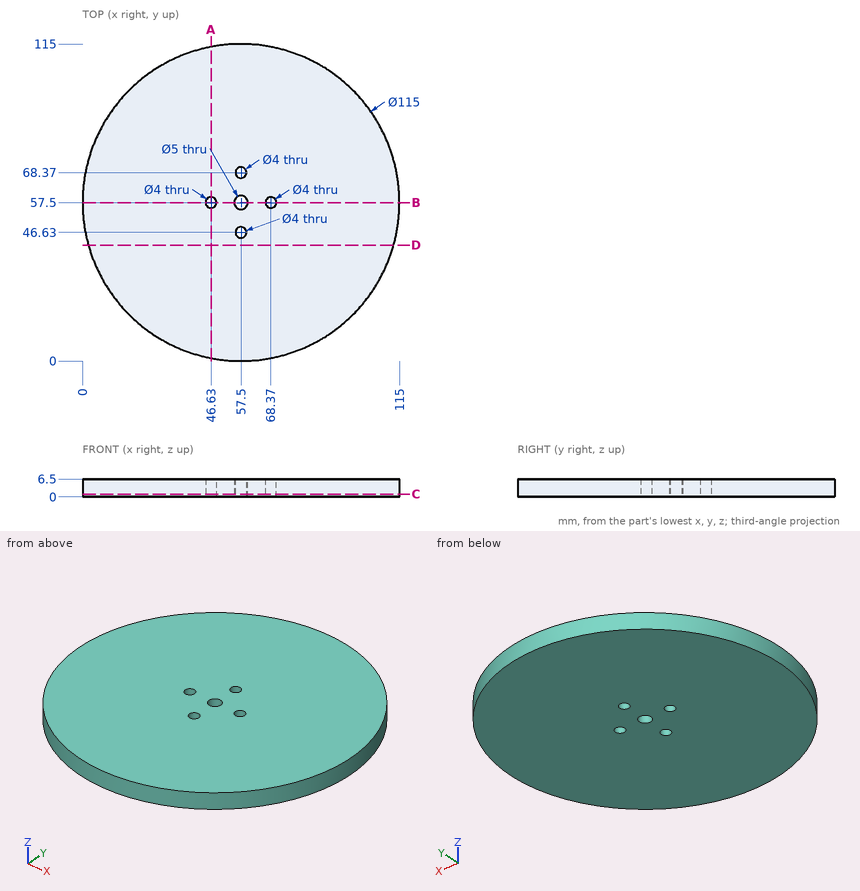
Job drawing, mm, ordinate dimensions from the low corner. One solid piece. Give positions to 0.01 mm unless a question says otherwise; leave off trailing zeros. Order: outer loops, then holes, each group sorted by start corner. A loop starts at its lowest first (then second) coordinate and runs counter-clockwise, first axis right, second up. Notation, with made-up numbers: (37, 58) -> (93, 58) arc R11 ccw to (93, 67) -> close; hole circle Ø10 at (74.25, 2.25). An arc over 180 degrees is marked (long way). Return JSON: item names as keys, results as strings.
Q1. Saw through at C-C (z = 1). Write the cut outline in (x, y).
Working result:
{"outline": "circle Ø115 at (57.5, 57.5); hole circle Ø4 at (46.63, 57.5); hole circle Ø5 at (57.5, 57.5); hole circle Ø4 at (57.5, 46.63); hole circle Ø4 at (57.5, 68.37); hole circle Ø4 at (68.37, 57.5)"}
Q2. Saw through at B-B (y = 57.5). Write the cut outline in (x, z), then the cut area to 3 significant figures.
Working result:
{"outline": "(0, 0) -> (44.63, 0) -> (44.63, 6.5) -> (0, 6.5) -> close; (48.63, 0) -> (55, 0) -> (55, 6.5) -> (48.63, 6.5) -> close; (60, 0) -> (66.37, 0) -> (66.37, 6.5) -> (60, 6.5) -> close; (70.37, 0) -> (115, 0) -> (115, 6.5) -> (70.37, 6.5) -> close", "area": "663 mm²"}
Q3. Flat gauge pin, fed straight in: pin 1 (2.5 mm diameter, centred on x = 57.5, y = 68.37, fed in from +Z). Where does the tip first touch, or does it go through?
Working result:
{"pin 1": "through"}
Q4. Saw through at D-D (y = 42). Write the cut outline in (x, z), then the cut area to 3 significant figures.
Working result:
{"outline": "(2.13, 0) -> (112.87, 0) -> (112.87, 6.5) -> (2.13, 6.5) -> close", "area": "720 mm²"}
Q5. Saw through at A-A (x = 46.63). Write the cut outline in (y, z).
Working result:
{"outline": "(1.04, 0) -> (55.5, 0) -> (55.5, 6.5) -> (1.04, 6.5) -> close; (59.5, 0) -> (113.96, 0) -> (113.96, 6.5) -> (59.5, 6.5) -> close"}
Q6. Drill centre lines: line 1 (Y direction, x = 57.5, z = 4.25); line 2 (X direction, y = 58.5, z = 5.75); line 3 (X direction, y = 58, z = 3). Where is each one in solid material? Low to high.
Working result:
{"line 1": "0 to 44.63, 48.63 to 55, 60 to 66.37, 70.37 to 115", "line 2": "0.01 to 44.9, 48.36 to 55.21, 59.79 to 66.64, 70.1 to 114.99", "line 3": "0 to 44.69, 48.57 to 55.05, 59.95 to 66.43, 70.31 to 115"}
